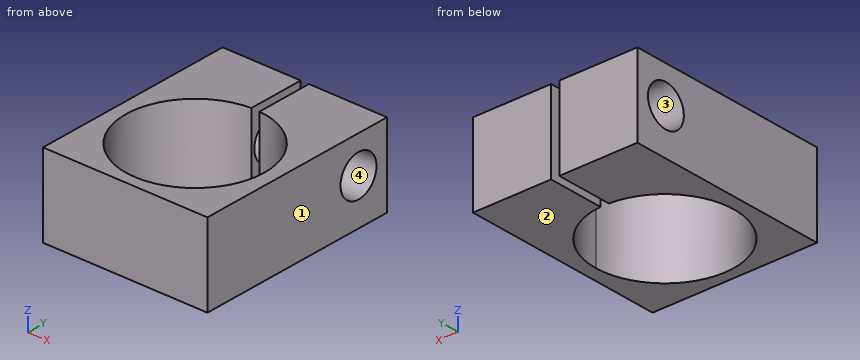
```python
from build123d import *

# Parameters (mm, degrees)
F0_W     = 20
F0_H     = 25
F0_R     = 8.4
F1_DEPTH = 10
F2_W     = 1
F2_H     = 6.8792646822
F3_DEPTH = 10
F4_R     = 2.5
F5_DEPTH = 20


with BuildPart() as f1:
    # F0 (on Top) → F1 (new body)
    with BuildSketch(Plane.XY):
        Rectangle(F0_W, F0_H)
        with Locations((0, -2.7643705253)):
            Circle(F0_R, mode=Mode.SUBTRACT)
    extrude(amount=F1_DEPTH)

    # F2 (on face) → F3 (cut)
    with BuildSketch(Plane.XY.offset(10)):
        with Locations((0, 9.0603676589)):
            Rectangle(F2_W, F2_H)
    extrude(amount=-F3_DEPTH, mode=Mode.SUBTRACT)

    # F4 (on face) → F5 (cut)
    with BuildSketch(Plane(origin=(-10, 0, 0), x_dir=(0, -1, 0), z_dir=(-1, 0, 0))):
        with Locations((-8.5356631532, 5.5329478068)):
            Circle(F4_R)
    extrude(amount=-F5_DEPTH, mode=Mode.SUBTRACT)


solid = f1.part
```
Design review of the part built by this model. Coordinates are the model's own, in mm. Face numbers are marked on the shaded views. Coordinates: 2 decimals unless noted, no trailing zeros. Write each loop counter-clockwise with the first axis right and the second up, starting at its lowest first coordinate (ties: lowest second). Pieces come first, ordered by that corner, then holes.
1) Add section A-A (x = -4.25). Write out the cut boundary in (y, z).
2) To check wall thickness, follow L1, parallel to X at y = 7, z = 8.25; L2, parallel to Y at x = 7.5, z = 7.5; L3, parallel to Y at x = -1.75, z = 6.5. State the ranges of each line that lie inside material, in increasing order.
3) Add section D-D (z = 2). Write out the cut boundary in (x, y).
4) Mouldability with a two-part tool opening along Z and no side actions: class the marked faces 1, 2, 3 and 4 as +Z half, -Z half, draft (parallel to the pull), parting line (faces both ways), or undercut.
5) Add section B-B (z = 7.75). Write out the cut boundary in (x, y), plus the area to 3 significant figures.
6) Add section C-C (y = 0.75). Write out the cut boundary in (x, z).
Check result:
1. outline: (-12.5, 0) - (-10.01, 0) - (-10.01, 10) - (-12.5, 10) - close; (4.48, 0) - (12.5, 0) - (12.5, 10) - (4.48, 10) - close; hole circle Ø5 at (8.54, 5.53)
2. L1: x = -10 to -0.5, 0.5 to 10
2. L2: y = -12.5 to -6.55, 1.02 to 6.99, 10.08 to 12.5
2. L3: y = -12.5 to -10.98, 5.45 to 6.23, 10.84 to 12.5
3. outline: (-10, -12.5) - (10, -12.5) - (10, 12.5) - (0.5, 12.5) - (0.5, 5.62) arc R8.4 cw (long way) to (-0.5, 5.62) - (-0.5, 12.5) - (-10, 12.5) - close
4. face 1: draft
4. face 2: -Z half
4. face 3: undercut
4. face 4: undercut
5. outline: (-10, -12.5) - (10, -12.5) - (10, 7.38) - (0.5, 7.38) - (0.5, 5.62) arc R8.4 cw (long way) to (-0.5, 5.62) - (-0.5, 7.38) - (-10, 7.38) - close; (-10, 9.69) - (-0.5, 9.69) - (-0.5, 12.5) - (-10, 12.5) - close; (0.5, 9.69) - (10, 9.69) - (10, 12.5) - (0.5, 12.5) - close
5. area: 228 mm2
6. outline: (-10, 0) - (-7.63, 0) - (-7.63, 10) - (-10, 10) - close; (7.63, 0) - (10, 0) - (10, 10) - (7.63, 10) - close
